For this review, take the finished solid that the model builds, in its own axes (mm). Coordinates: 2 decimals unless noted, no trailing zeros. Write each loop counter-clockwise with the first axis right and the second up, starting at its lowest first coordinate (ties: lowest second). Pieces come first, ordered by that corner, then holes.
```python
from build123d import *

# Parameters (mm, degrees)
GRUNDFORM_DEPTH = 28


with BuildPart() as part:
    # Skizze2 → Grundform (new body)
    with BuildSketch(Plane.XY):
        with BuildLine():
            ThreePointArc((54.076028974, 45.058183854), (0, 47.5), (-54.076028974, 45.058183854))
            ThreePointArc((-54.076028974, 45.058183854), (-63.534180091, 40.5184013), (-67.704234102, 30.891517187))
            ThreePointArc((-67.704234102, 30.891517187), (-68.5, 0), (-67.704234102, -30.891517187))
            ThreePointArc((-67.704234102, -30.891517187), (-63.534180091, -40.5184013), (-54.076028974, -45.058183854))
            ThreePointArc((-54.076028974, -45.058183854), (0, -47.5), (54.076028974, -45.058183854))
            ThreePointArc((54.076028974, -45.058183854), (63.534180091, -40.5184013), (67.704234102, -30.891517187))
            ThreePointArc((67.704234102, -30.891517187), (68.5, 0), (67.704234102, 30.891517187))
            ThreePointArc((67.704234102, 30.891517187), (63.534180091, 40.5184013), (54.076028974, 45.058183854))
        make_face()
    extrude(amount=GRUNDFORM_DEPTH)


solid = part.part
```
Q1. Add section B-B (x = 42). State the section outline as (y, z) points.
Ans:
outline: (-46.03, 0) - (46.03, 0) - (46.03, 28) - (-46.03, 28) - close
Q2. Add section A-A (z = 10). State the section outline as (x, y) points.
Ans:
outline: (-67.7, -30.89) arc R15 ccw to (-54.08, -45.06) arc R600 ccw to (54.08, -45.06) arc R15 ccw to (67.7, -30.89) arc R600 ccw to (67.7, 30.89) arc R15 ccw to (54.08, 45.06) arc R600 ccw to (-54.08, 45.06) arc R15 ccw to (-67.7, 30.89) arc R600 ccw to start
Q3. Clearance check with flat-ended pins moving along their axes: pin 1 Ø10 at (x, z) = (-11, 13) entering from -Y; pin 2 Ø5 at (x, y) = (-7.5, -36) entering from -Z; pin 3 Ø2 at (x, z) = (10, 11.5) entering from +Y; pin 4 Ø4 at (y, z) = (29, 6) entering from +X. State where each tip first meets the part, or that it passes through.
Ans:
pin 1: stops at y = -47.47
pin 2: stops at z = 0
pin 3: stops at y = 47.43
pin 4: stops at x = 67.89
Q4. For probe 1 along X at (y, z) = (1.5, 10); probe 2 along Y at (x, z) = (1, 9.75); probe 3 along X at (y, z) = (30.5, 9), list the stretches that pass through material, from the lowest coordinate up.
Ans:
probe 1: x = -68.5 to 68.5
probe 2: y = -47.5 to 47.5
probe 3: x = -67.72 to 67.72
